```python
from build123d import *

# Parameters (mm, degrees)
SKETCH1_W                                           = 10
SKETCH1_H                                           = 100
BOSS_EXTRUDE1_DEPTH                                 = 50
SKETCH2_R                                           = 42
CUT_EXTRUDE1_DEPTH                                  = 4
CUT_EXTRUDE3_REACH                                  = 72.965
SKETCH4_R                                           = 22.75
M3_TAPPED_HOLE1_D                                   = 2.5
FILLET3_R                                           = 0.5
CHAMFER1_SIZE                                       = 1
CBORE_FOR_M4_HEX_SOCKET_HEAD_CAP_SCREW1_D           = 4.5
CBORE_FOR_M4_HEX_SOCKET_HEAD_CAP_SCREW1_CBORE_D     = 8
CBORE_FOR_M4_HEX_SOCKET_HEAD_CAP_SCREW1_CBORE_DEPTH = 5
M4_TAPPED_HOLE1_D                                   = 3.3
M4_TAPPED_HOLE1_DEPTH                               = 11
M4_TAPPED_HOLE1_TIP                                 = 0.991420021
M4_TAPPED_HOLE2_D                                   = 3.3
M4_TAPPED_HOLE2_DEPTH                               = 11
M4_TAPPED_HOLE2_TIP                                 = 0.991420021
M4_TAPPED_HOLE3_D                                   = 3.3
M4_TAPPED_HOLE3_DEPTH                               = 11
M4_TAPPED_HOLE3_TIP                                 = 0.991420021
M4_TAPPED_HOLE4_D                                   = 3.3


with BuildPart() as part:
    # Sketch1 → Boss-Extrude1 (new, symmetric)
    with BuildSketch(Plane(origin=(0, 0, 0), x_dir=(0, 0, -1), z_dir=(1, 0, 0))):
        Rectangle(SKETCH1_W, SKETCH1_H)
    extrude(amount=BOSS_EXTRUDE1_DEPTH, both=True)

    # Sketch2 → Cut-Extrude1 (cut)
    with BuildSketch(Plane.XY.offset(5)):
        Circle(SKETCH2_R)
    extrude(amount=-CUT_EXTRUDE1_DEPTH, mode=Mode.SUBTRACT)

    # Sketch4 → Cut-Extrude3 (cut, up to next)
    with BuildSketch(Plane.XY.offset(1), mode=Mode.PRIVATE) as cut_extrude3_sk1:
        Circle(SKETCH4_R)
    cut_extrude3_tool1 = extrude(cut_extrude3_sk1.sketch, amount=-CUT_EXTRUDE3_REACH, mode=Mode.PRIVATE) & part.part
    add(cut_extrude3_tool1.solids().sort_by_distance((0, 0, 1))[0], mode=Mode.SUBTRACT)

    # M3 Tapped Hole1 (through all)
    with Locations(Plane.XY.offset(1)):
        with Locations((-32.04293994, -18.5), (-37, 0), (37, 0), (18.5, 32.04293994), (-32.04293994, 18.5), (32.04293994, -18.5), (-18.5, -32.04293994), (0, 37), (0, -37), (-18.5, 32.04293994), (18.5, -32.04293994), (32.04293994, 18.5)):
            Hole(M3_TAPPED_HOLE1_D / 2)

    # Fillet3
    fillet3_edges = [part.edges().sort_by_distance(p)[0] for p in [
        (-42, 0, 1),
    ]]
    fillet(fillet3_edges, radius=FILLET3_R)

    # Chamfer1
    chamfer1_edges = [part.edges().sort_by_distance(p)[0] for p in [
        (-42, 0, 5),
        (-22.75, 0, 1),
    ]]
    chamfer(chamfer1_edges, length=CHAMFER1_SIZE)

    # CBORE for M4 Hex Socket Head Cap Screw1 (through all)
    with Locations(Plane.XY.offset(5)):
        with Locations((-45, -45), (-25, -45), (25, -45), (45, -45)):
            CounterBoreHole(CBORE_FOR_M4_HEX_SOCKET_HEAD_CAP_SCREW1_D / 2, CBORE_FOR_M4_HEX_SOCKET_HEAD_CAP_SCREW1_CBORE_D / 2, CBORE_FOR_M4_HEX_SOCKET_HEAD_CAP_SCREW1_CBORE_DEPTH)

    # M4 Tapped Hole1
    with Locations(Plane(origin=(0, 50, 0), x_dir=(1, 0, 0), z_dir=(0, 1, 0))):
        with Locations((-45, 0), (-25, 0), (25, 0), (45, 0)):
            Hole(M4_TAPPED_HOLE1_D / 2, depth=M4_TAPPED_HOLE1_DEPTH)
            with Locations((0, 0, -(M4_TAPPED_HOLE1_DEPTH + M4_TAPPED_HOLE1_TIP / 2))):  # 118° drill point
                Cone(0, M4_TAPPED_HOLE1_D / 2, M4_TAPPED_HOLE1_TIP, mode=Mode.SUBTRACT)

    # M4 Tapped Hole2
    with Locations(Plane(origin=(50, 0, 0), x_dir=(0, 0, -1), z_dir=(1, 0, 0))):
        with Locations((0, 25), (0, -25)):
            Hole(M4_TAPPED_HOLE2_D / 2, depth=M4_TAPPED_HOLE2_DEPTH)
            with Locations((0, 0, -(M4_TAPPED_HOLE2_DEPTH + M4_TAPPED_HOLE2_TIP / 2))):  # 118° drill point
                Cone(0, M4_TAPPED_HOLE2_D / 2, M4_TAPPED_HOLE2_TIP, mode=Mode.SUBTRACT)

    # M4 Tapped Hole3
    with Locations(Plane.ZY.offset(50)):
        with Locations((0, 25), (0, -25)):
            Hole(M4_TAPPED_HOLE3_D / 2, depth=M4_TAPPED_HOLE3_DEPTH)
            with Locations((0, 0, -(M4_TAPPED_HOLE3_DEPTH + M4_TAPPED_HOLE3_TIP / 2))):  # 118° drill point
                Cone(0, M4_TAPPED_HOLE3_D / 2, M4_TAPPED_HOLE3_TIP, mode=Mode.SUBTRACT)

    # M4 Tapped Hole4 (through all)
    with Locations(Plane.XY.offset(5)):
        with Locations((35.355339059, -35.355339059), (35.355339059, 35.355339059), (-35.355339059, 35.355339059), (-35.355339059, -35.355339059)):
            Hole(M4_TAPPED_HOLE4_D / 2)


solid = part.part
```
Design review of the part built by this model. Coordinates are the model's own, in mm. A direction names the side the tool comes from. Give positions to 0.01 mm unless a question says otherwise; leave off trailing zeros. One line per item, written item: value.
Q1. Draft analysis for pull direction X (two halves, no side actions). For faces 1 (the cylindrical face through (-26.21, -43.103, -2.535)), 2 (the cylindrical face through (-44.423, 26.636, 0.215)), 3 (the conical face through (-38.18, 25.28, -0.04)), state which applies: pulls with the +X half, pulls with the -X half, needs draft (parallel to the pull), parting line crosses it, or undercut.
Numbers:
face 1: undercut
face 2: needs draft
face 3: pulls with the -X half
Q2. We need section A-A on y = -18.5. Give the number of separate pieces and of enclosed holes in the cut face, and give its area (3 significant figures).
Numbers:
separate pieces: 4
enclosed holes: 0
area: 507 mm^2
Q3. Machinability: for faces 4 (the cylindrical face through (40.06, 12.62, 2.77)), 5 (the cylindrical face through (30.89, -18.98, -2.04)), 6 (the cylindrical face through (46.65, 44.42, -0.07)), which of the approach directions +Z, -Z, +X, -X, +Y, -Y give a long, thin tool a straight path to every point of the face, cutting with its end or side? Answer none if there is none.
Numbers:
face 4: +Z
face 5: +Z, -Z
face 6: +Y
Q4. For L1, parallel to Y at x = 0, z = -1.7; L2, parallel to Y at x = 39.5, z = 0.25; L3, parallel to Y at x = 25, z = -2.15, list the stretches that pass through material, from the lowest coordinate up.
Numbers:
L1: y = -50 to -38.25, -35.75 to -22.75, 22.75 to 35.75, 38.25 to 50
L2: y = -50 to -26.63, -23.37 to 23.37, 26.63 to 50
L3: y = -50 to -47.25, -42.75 to 50
Q5. For pin 1 Ø1.5 at (x, y) = (7.5, 19) entering from -Z; pin 2 Ø7 at (x, y) = (-25, -45) entering from +Z; pin 3 Ø2.5 at (y, z) = (-25, 0) entering from +X; pin 4 Ø2 at (x, y) = (-8, 25.5) entering from +Z, all flat-tipped, find the tip position at first contact; note any pin that passes through.
Numbers:
pin 1: passes through
pin 2: stops at z = 0
pin 3: stops at x = 38.76
pin 4: stops at z = 1
